Source: CAD feature listing. Evaluate the final solid. Frame: model axes, mm. A direction names the side the tool comes from. Coordinates: 2 decimals unless noted, no trailing zeros. Loops run counter-clockwise (first coordinate to the right, second up) from the corner with the lowest first, then second, coordinate; pieces in that order, holes last. Notation, with made-up numbers: (-12.75, 3) -> (33.25, 3) arc R10 ccw to (33.25, 11) -> close; hole circle Ø10 at (40.25, -33). An arc over 180 degrees is marked (long way). Answer as CSV lines item,"result".
from build123d import *

# Parameters (mm, degrees)
SALIENTE_EXTRUIR1_DEPTH = 1.5
SALIENTE_EXTRUIR3_DEPTH = 13
CROQUIS4_W              = 15
CROQUIS4_H              = 1.5
CROQUIS4_H_2            = 2
SALIENTE_EXTRUIR4_DEPTH = 5
CROQUIS5_W              = 1.5
CROQUIS5_H              = 10
CROQUIS5_W_2            = 1.75
SALIENTE_EXTRUIR5_DEPTH = 2.5
CROQUIS6_W              = 18.5
CROQUIS6_H              = 7
CORTAR_EXTRUIR1_DEPTH   = 1.5
CROQUIS7_W              = 10
CROQUIS7_H              = 4.5
CORTAR_EXTRUIR2_DEPTH   = 1.5
CROQUIS8_R              = 2.25
CROQUIS8_R_2            = 1.5
SALIENTE_EXTRUIR6_DEPTH = 2.25
CORTAR_EXTRUIR3_REACH   = 56.695
CROQUIS9_R              = 1.75
CROQUIS10_R             = 2.125
CORTAR_EXTRUIR4_DEPTH   = 1.5
CROQUIS11_R             = 2.125
CORTAR_EXTRUIR5_DEPTH   = 1.5
SALIENTE_EXTRUIR8_DEPTH = 1.5
SALIENTE_EXTRUIR9_DEPTH = 1.5
REDONDEO2_R             = 2


with BuildPart() as part:
    # Croquis1 → Saliente-Extruir1 (new body)
    with BuildSketch(Plane(origin=(0, 0, 0), x_dir=(1, 0, 0), z_dir=(0, 1, 0))):
        with BuildLine():
            Line((-25.5, -22.5), (25.5, -22.5))
            ThreePointArc((25.5, -22.5), (26.914213562, -21.914213562), (27.5, -20.5))
            Line((27.5, -20.5), (27.5, 20.5))
            ThreePointArc((27.5, 20.5), (26.914213562, 21.914213562), (25.5, 22.5))
            Line((25.5, 22.5), (-25.5, 22.5))
            ThreePointArc((-25.5, 22.5), (-26.914213562, 21.914213562), (-27.5, 20.5))
            Line((-27.5, 20.5), (-27.5, -20.5))
            ThreePointArc((-27.5, -20.5), (-26.914213562, -21.914213562), (-25.5, -22.5))
        make_face()
    extrude(amount=SALIENTE_EXTRUIR1_DEPTH)

    # Croquis3 → Saliente-Extruir3 (add)
    with BuildSketch(Plane(origin=(0, 1.5, 0), x_dir=(1, 0, 0), z_dir=(0, 1, 0))):
        with BuildLine():
            Line((-25.5, 22.5), (25.5, 22.5))
            ThreePointArc((25.5, 22.5), (26.914213562, 21.914213562), (27.5, 20.5))
            Line((27.5, 20.5), (27.5, -20.5))
            ThreePointArc((27.5, -20.5), (26.914213562, -21.914213562), (25.5, -22.5))
            Line((25.5, -22.5), (-25.5, -22.5))
            ThreePointArc((-25.5, -22.5), (-26.914213562, -21.914213562), (-27.5, -20.5))
            Line((-27.5, -20.5), (-27.5, 20.5))
            ThreePointArc((-27.5, 20.5), (-26.914213562, 21.914213562), (-25.5, 22.5))
        make_face()
        with BuildLine():
            Line((-25.5, 21), (25.5, 21))
            ThreePointArc((25.5, 21), (25.853553391, 20.853553391), (26, 20.5))
            Line((26, 20.5), (26, -20.5))
            ThreePointArc((26, -20.5), (25.853553391, -20.853553391), (25.5, -21))
            Line((25.5, -21), (-25.5, -21))
            ThreePointArc((-25.5, -21), (-25.853553391, -20.853553391), (-26, -20.5))
            Line((-26, -20.5), (-26, 20.5))
            ThreePointArc((-26, 20.5), (-25.853553391, 20.853553391), (-25.5, 21))
        make_face(mode=Mode.SUBTRACT)
    extrude(amount=SALIENTE_EXTRUIR3_DEPTH)

    # Croquis4 → Saliente-Extruir4 (add)
    with BuildSketch(Plane(origin=(0, 1.5, 0), x_dir=(1, 0, 0), z_dir=(0, 1, 0))):
        with Locations((-6, 19.25)):
            Rectangle(CROQUIS4_W, CROQUIS4_H)
        with Locations((-6, -19.25)):
            Rectangle(CROQUIS4_W, CROQUIS4_H)
        with Locations((-3.5, 0.675)):
            Rectangle(CROQUIS4_W, CROQUIS4_H_2)
    extrude(amount=SALIENTE_EXTRUIR4_DEPTH)

    # Croquis5 → Saliente-Extruir5 (add)
    with BuildSketch(Plane(origin=(0, 1.5, 0), x_dir=(1, 0, 0), z_dir=(0, 1, 0))):
        with Locations((12.75, 10)):
            Rectangle(CROQUIS5_W, CROQUIS5_H)
        with Locations((8.875, -9.25)):
            Rectangle(CROQUIS5_W_2, CROQUIS5_H)
    extrude(amount=SALIENTE_EXTRUIR5_DEPTH)

    # Croquis6 → Cortar-Extruir1 (cut)
    with BuildSketch(Plane.ZY.offset(27.5)):
        with Locations((9.25, 11)):
            Rectangle(CROQUIS6_W, CROQUIS6_H)
    extrude(amount=-CORTAR_EXTRUIR1_DEPTH, mode=Mode.SUBTRACT)

    # Croquis7 → Cortar-Extruir2 (cut)
    with BuildSketch(Plane.XY.offset(22.5)):
        with Locations((-8.5, 12.25)):
            Rectangle(CROQUIS7_W, CROQUIS7_H)
    extrude(amount=-CORTAR_EXTRUIR2_DEPTH, mode=Mode.SUBTRACT)

    # Croquis8 → Saliente-Extruir6 (add)
    # profile 1 of 2: a face of its own
    with BuildSketch(Plane(origin=(0, 1.5, 0), x_dir=(1, 0, 0), z_dir=(0, 1, 0))):
        with Locations(Location((23, -18, 0), (0, 0, 270))):
            Circle(CROQUIS8_R)
        with Locations(Location((23, -18, 0), (0, 0, 270))):
            Circle(CROQUIS8_R_2, mode=Mode.SUBTRACT)
    # profile 2 of 2: a face of its own
    with BuildSketch(Plane(origin=(0, 1.5, 0), x_dir=(1, 0, 0), z_dir=(0, 1, 0))):
        with Locations(Location((23, -0.5, 0), (0, 0, 270))):
            Circle(CROQUIS8_R)
        with Locations(Location((23, -0.5, 0), (0, 0, 270))):
            Circle(CROQUIS8_R_2, mode=Mode.SUBTRACT)
    extrude(amount=SALIENTE_EXTRUIR6_DEPTH)

    # Cortar-Extruir3: up to this face of the body (flat: up to its plane)
    cortar_extruir3_end = Plane(part.part.faces().sort_by_distance((0.55075594, 6.926025918, 22.5))[0])
    # Croquis9 → Cortar-Extruir3 (cut, up to the picked face)
    with BuildSketch(Plane(origin=(0, 0, -22.5), x_dir=(-1, 0, 0), z_dir=(0, 0, -1)), mode=Mode.PRIVATE) as cortar_extruir3_sk1:
        with Locations((0, 10)):
            Circle(CROQUIS9_R)
    cortar_extruir3_tool1 = split(extrude(cortar_extruir3_sk1.sketch, amount=-CORTAR_EXTRUIR3_REACH, mode=Mode.PRIVATE), bisect_by=cortar_extruir3_end, keep=Keep.BOTH, mode=Mode.PRIVATE)
    add(cortar_extruir3_tool1.solids().sort_by(Axis((0, 10, -22.5), (0, 0, 1)))[0], mode=Mode.SUBTRACT)

    # Croquis10 → Cortar-Extruir4 (cut)
    with BuildSketch(Plane(origin=(0, 1.5, 0), x_dir=(1, 0, 0), z_dir=(0, 1, 0))):
        with Locations(Location((-16, 0, 0), (0, 0, 270))):
            Circle(CROQUIS10_R)
        with Locations(Location((16, 0, 0), (0, 0, 270))):
            Circle(CROQUIS10_R)
    extrude(amount=-CORTAR_EXTRUIR4_DEPTH, mode=Mode.SUBTRACT)

    # Croquis11 → Cortar-Extruir5 (cut)
    with BuildSketch(Plane(origin=(0, 1.5, 0), x_dir=(1, 0, 0), z_dir=(0, 1, 0))):
        with Locations(Location((-20, 12, 0), (0, 0, 270))):
            Circle(CROQUIS11_R)
        with Locations(Location((20, 12, 0), (0, 0, 270))):
            Circle(CROQUIS11_R)
        with Locations(Location((20, -12, 0), (0, 0, 270))):
            Circle(CROQUIS11_R)
        with Locations(Location((-20, -12, 0), (0, 0, 270))):
            Circle(CROQUIS11_R)
    extrude(amount=-CORTAR_EXTRUIR5_DEPTH, mode=Mode.SUBTRACT)

    # Croquis12 → Saliente-Extruir8 (add)
    with BuildSketch(Plane.ZY.offset(27.5)):
        with BuildLine():
            Line((0, 7.5), (2, 7.5))
            ThreePointArc((2, 7.5), (0.585786438, 8.085786438), (0, 9.5))
            Line((0, 9.5), (0, 7.5))
        make_face()
        with BuildLine():
            Line((18.5, 9.5), (18.5, 7.5))
            Line((18.5, 7.5), (16.5, 7.5))
            ThreePointArc((16.5, 7.5), (17.914213562, 8.085786438), (18.5, 9.5))
        make_face()
    extrude(amount=-SALIENTE_EXTRUIR8_DEPTH)

    # Croquis13 → Saliente-Extruir9 (add)
    with BuildSketch(Plane.XY.offset(22.5)):
        with BuildLine():
            Line((-13.5, 12), (-13.5, 10))
            Line((-13.5, 10), (-11.5, 10))
            ThreePointArc((-11.5, 10), (-12.914213562, 10.585786438), (-13.5, 12))
        make_face()
        with BuildLine():
            Line((-3.5, 12), (-3.5, 10))
            Line((-3.5, 10), (-5.5, 10))
            ThreePointArc((-5.5, 10), (-4.085786438, 10.585786438), (-3.5, 12))
        make_face()
    extrude(amount=-SALIENTE_EXTRUIR9_DEPTH)

    # Redondeo2
    redondeo2_edges = [part.edges().sort_by_distance(p)[0] for p in [
        (12.75, 4, -15),
        (12.75, 4, -5),
        (8.875, 4, 4.25),
        (8.875, 4, 14.25),
        (-13.5, 6.5, -19.25),
        (1.5, 6.5, -19.25),
        (1.5, 6.5, 19.25),
        (-13.5, 6.5, 19.25),
        (-11, 6.5, -0.675),
        (4, 6.5, -0.675),
    ]]
    fillet(redondeo2_edges, radius=REDONDEO2_R)


solid = part.part
(1) Cut plane C-C (z = -12). Return the cut outline in (x, y) (3 decimals).
Computed values:
outline,"(-27.5, 0) -> (-22.125, 0) -> (-22.125, 1.5) -> (-26, 1.5) -> (-26, 14.5) -> (-27.5, 14.5) -> close; (-17.875, 0) -> (17.875, 0) -> (17.875, 1.5) -> (13.5, 1.5) -> (13.5, 4) -> (12, 4) -> (12, 1.5) -> (-17.875, 1.5) -> close; (22.125, 0) -> (27.5, 0) -> (27.5, 14.5) -> (26, 14.5) -> (26, 1.5) -> (22.125, 1.5) -> close"
(2) Draft query along X for faces 3 (the flat face through (-27, 12, 0)), 4 (the cylindrical face through (26.9, 7.15, -21.93)), 5 (the flat face through (1.5, 3, 19)). Return one class per face: released by +X, released by -X, zero draft, split by the parting line, or undercut.
Computed values:
face 3,"zero draft"
face 4,"released by +X"
face 5,"undercut"
(3) Cut plane B-B (x = -20). Return the cut outline in (y, z) (3 decimals).
Computed values:
outline,"(0, -22.5) -> (14.5, -22.5) -> (14.5, -21) -> (1.5, -21) -> (1.5, -14.125) -> (0, -14.125) -> close; (0, -9.875) -> (1.5, -9.875) -> (1.5, 9.875) -> (0, 9.875) -> close; (0, 14.125) -> (1.5, 14.125) -> (1.5, 21) -> (14.5, 21) -> (14.5, 22.5) -> (0, 22.5) -> close"
(4) Material intervals for L1, parallel to X at y = 0.3, z = 12 (3 decimals); L2, parallel to X at y = 3.15, z = 18; L3, parallel to X at y = 0.3, z = 0 (3 decimals), sorted ascending. Write a range as [from, to].
Computed values:
L1,"[-27.5, -22.125], [-17.875, 17.875], [22.125, 27.5]"
L2,"[-27.5, -26], [20.75, 21.5], [24.5, 25.25], [26, 27.5]"
L3,"[-27.5, -18.125], [-13.875, 13.875], [18.125, 27.5]"
(5) Cut plane A-A (y = 13.75). Return the cut outline in (x, z), then the cut area to 3 significant figures.
Computed values:
outline,"(-27.5, -20.5) arc R2 ccw to (-25.5, -22.5) -> (25.5, -22.5) arc R2 ccw to (27.5, -20.5) -> (27.5, 20.5) arc R2 ccw to (25.5, 22.5) -> (-3.5, 22.5) -> (-3.5, 21) -> (25.5, 21) arc R0.5 cw to (26, 20.5) -> (26, -20.5) arc R0.5 cw to (25.5, -21) -> (-25.5, -21) arc R0.5 cw to (-26, -20.5) -> (-26, 0) -> (-27.5, 0) -> close; (-27.5, 18.5) -> (-26, 18.5) -> (-26, 20.5) arc R0.5 cw to (-25.5, 21) -> (-13.5, 21) -> (-13.5, 22.5) -> (-25.5, 22.5) arc R2 ccw to (-27.5, 20.5) -> close"
area,"245 mm^2"
(6) Pin query (flat end, axial travel): pin 1 Ø6 at (x, z) = (2, 16) entering from +Y; pin 2 Ø3 at (x, z) = (2.5, 1) entering from -Y; pin 3 Ø12.5 at (x, z) = (6.5, -6) entering from +Y; pin 4 Ø1.6 at (x, z) = (-8.5, 21.5) entering from +Y. Return the tip coordinate at first contact, or that it passes through.
Computed values:
pin 1,"y = 6.31"
pin 2,"y = 0"
pin 3,"y = 6.5"
pin 4,"y = 10"
(7) Cut plane D-D (x = 23). Return the cut outline in (y, z).
Computed values:
outline,"(0, -22.5) -> (14.5, -22.5) -> (14.5, -21) -> (1.5, -21) -> (1.5, -1.75) -> (3.75, -1.75) -> (3.75, -1) -> (1.5, -1) -> (1.5, 2) -> (3.75, 2) -> (3.75, 2.75) -> (1.5, 2.75) -> (1.5, 15.75) -> (3.75, 15.75) -> (3.75, 16.5) -> (1.5, 16.5) -> (1.5, 19.5) -> (3.75, 19.5) -> (3.75, 20.25) -> (1.5, 20.25) -> (1.5, 21) -> (14.5, 21) -> (14.5, 22.5) -> (0, 22.5) -> close"
(8) Access query for faces 1 (the cylindrical face through (-12.9, 10.57, 21.76)), 2 (the flat face through (-4, 4, -1.675)). Directions: +Z, -Z, +X, -X, +Y, -Y. A direction counts if a zero-diameter tool reaches every point of the face in a straight line with its end or side. Return the directions, or none.
Computed values:
face 1,"+Z, +Y"
face 2,"+Y"
